Build history of the part. All positions in model axes, mm. A direction names the side the tool comes from. Round coordinates to 2 decimals unless told otherwise and drop trailing zeros. Write each loop counter-clockwise with the first axis right and the second up, starting at its lowest first coordinate (ties: lowest second). Pieces come first, ordered by that corner, then holes.
from build123d import *

# Parameters (mm, degrees)
SKETCH1_W           = 30
SKETCH1_H           = 85
BOSS_EXTRUDE1_DEPTH = 7
SKETCH2_W           = 4.15
SKETCH2_H           = 23.15
CUT_EXTRUDE1_DEPTH  = 8
SKETCH3_R           = 2.25
CUT_EXTRUDE2_DEPTH  = 8
CHAMFER1_SIZE       = 1


with BuildPart() as part:
    # Sketch1 → Boss-Extrude1 (new body)
    with BuildSketch(Plane(origin=(0, 0, 0), x_dir=(1, 0, 0), z_dir=(0, 1, 0))):
        with Locations((15, 42.5)):
            Rectangle(SKETCH1_W, SKETCH1_H)
    extrude(amount=BOSS_EXTRUDE1_DEPTH)

    # Sketch2 → Cut-Extrude1 (cut, through all)
    with BuildSketch(Plane(origin=(0, 7, 0), x_dir=(1, 0, 0), z_dir=(0, 1, 0))):
        with Locations((2.075, 42.5)):
            Rectangle(SKETCH2_W, SKETCH2_H)
        with Locations((27.925, 42.5)):
            Rectangle(SKETCH2_W, SKETCH2_H)
    extrude(amount=-CUT_EXTRUDE1_DEPTH, mode=Mode.SUBTRACT)

    # Sketch3 → Cut-Extrude2 (cut, through all)
    with BuildSketch(Plane(origin=(0, 7, 0), x_dir=(1, 0, 0), z_dir=(0, 1, 0))):
        with Locations((15, 49)):
            Circle(SKETCH3_R)
        with Locations((15, 36)):
            Circle(SKETCH3_R)
    extrude(amount=-CUT_EXTRUDE2_DEPTH, mode=Mode.SUBTRACT)

    # Chamfer1
    chamfer1_edges = [part.edges().sort_by_distance(p)[0] for p in [
        (12.75, 7, -49),
        (12.75, 7, -36),
    ]]
    chamfer(chamfer1_edges, length=CHAMFER1_SIZE)


solid = part.part
1) Slice it at A-A (z = -36). Write the cut outline in (x, y), plus the area to 3 significant figures.
Results:
outline: (4.15, 0) - (12.75, 0) - (12.75, 6) - (11.75, 7) - (4.15, 7) - close; (17.25, 0) - (25.85, 0) - (25.85, 7) - (18.25, 7) - (17.25, 6) - close
area: 119 mm2
2) Mould opens along Z. For faces 1 (the flat face through (2, 4, -30.925)), 2 (the flat face through (15, 3, -85)), 3 (the flat face through (0, 3, -69)) say: released by +Z, released by -Z, zero draft, split by the parting line, or undercut.
Results:
face 1: undercut
face 2: released by -Z
face 3: zero draft
3) Slice it at C-C (y = 2.5). Write the cut outline in (x, z) (3 decimals), plus the area to 3 significant figures.
Results:
outline: (0, -85) - (30, -85) - (30, -54.075) - (25.85, -54.075) - (25.85, -30.925) - (30, -30.925) - (30, 0) - (0, 0) - (0, -30.925) - (4.15, -30.925) - (4.15, -54.075) - (0, -54.075) - close; hole circle Ø4.5 at (15, -49); hole circle Ø4.5 at (15, -36)
area: 2,330 mm2
4) Slice it at B-B (x = 15). Write the cut outline in (y, z).
Results:
outline: (0, -85) - (7, -85) - (7, -52.25) - (6, -51.25) - (0, -51.25) - close; (0, -46.75) - (6, -46.75) - (7, -45.75) - (7, -39.25) - (6, -38.25) - (0, -38.25) - close; (0, -33.75) - (6, -33.75) - (7, -32.75) - (7, 0) - (0, 0) - close
5) Wall check: L1, parallel to Z at x = 15, y = 3.5; L2, parallel to X at y = 4.6, z = -36; L3, parallel to Z at x = 14.25, y = 5. Give the ranges that are in metal, low to high.
Results:
L1: z = -85 to -51.25, -46.75 to -38.25, -33.75 to 0
L2: x = 4.15 to 12.75, 17.25 to 25.85
L3: z = -85 to -51.12, -46.88 to -38.12, -33.88 to 0
6) Which spindle directions (+Z, -Z, +X, -X, +Y, -Y) get a long thin tool onto all of the face, cutting with end or side? Do faces 4 (the flat face through (25.85, 4, -42)), 5 (the flat face through (0, 3, -15)), 6 (the flat face through (4.15, 4, -42)). Say none if no direction does.
Results:
face 4: +X, +Y, -Y
face 5: +Z, -Z, -X, +Y, -Y
face 6: -X, +Y, -Y
7) Pin check, flat tips, straight feed: pin 1 Ø3 at (y, z) = (6, -11.5) entering from -X; pin 2 Ø2 at (y, z) = (6, -51.5) entering from +X; pin 3 Ø2 at (y, z) = (3.5, -41) entering from -X. Stop position of each tip, or through.
Results:
pin 1: stops at x = 0
pin 2: stops at x = 25.85
pin 3: stops at x = 4.15
